For this review, take the finished solid that the model builds, in its own axes (mm). A direction names the side the tool comes from. Coordinates: 2 decimals unless noted, no trailing zeros. Order: outer loops, then holes, each group sorted by start corner. A loop starts at its lowest first (then second) coordinate and runs counter-clockwise, first axis right, second up. Notation, with made-up numbers: M -38,87.25 L 20,87.25 A10 ccw 20,100.25 Z; hole C 5,44 d11. An arc over 180 degrees is marked long. Use one line per item in the form item = value. Start each with the question number.
Solid Edge part; units mm, degrees
sketch "Sketch1" plane through (0, 0, 0) normal (0, -1, 0) x (1, 0, 0)
  line L0 (0, 0) -> (-120, 0)
  line L1 (-120, 0) -> (-120, -10)
  line L2 (-120, -10) -> (-10, -10)
  line L3 (-10, -10) -> (-10, -60)
  line L4 (-10, -60) -> (0, -60)
  line L5 (0, -60) -> (0, 0)
extrude "Protrusion1" add sketch "Sketch1" along normal mid plane 60
sketch "Sketch2" plane through (-42.4264, 0, 42.4264) normal (0.7071068, 0, 0.7071068) x (0, -1, 0)
  line L0 (20, 60) -> (20, 20)
  line L1 (0, 60) -> (20, 60)
  line L2 (-20, 60) -> (0, 60)
  line L3 (-20, 20) -> (-20, 60)
  arc A0 (-20, 20) -> (20, 20) centre (0, 20) ccw
extrude "Protrusion2" add sketch "Sketch2" against normal up to next
sketch "Sketch3" plane through (-21.2132, 0, 21.2132) normal (0.7071068, 0, 0.7071068) x (0, 1, 0)
  circle A0 centre (0, 10.3051) radius 10
extrude "ExtrudedCutout_1" cut sketch "Sketch3" against normal blind 40
sketch "Sketch4" plane through (-28.2843, -20, 14.1421) normal (0, -1, 0) x (1, 0, 0)
  line L0 (10.1152, 4.0269) -> (3.0442, -3.0442)
  line L1 (3.0442, -3.0442) -> (10.1152, -10.1152)
  line L2 (10.1152, -10.1152) -> (17.1863, -3.0442)
  line L3 (17.1863, -3.0442) -> (10.1152, 4.0269)
extrude "Cutout1" cut sketch "Sketch4" against normal up to surface (40 mm away)
sketch "Sketch5" plane through (-60, 0, 0) normal (0, 0, 1) x (1, 0, 0)
  circle A0 centre (-50, -20) radius 5
extrude "Cutout2" cut sketch "Sketch5" against normal up to surface (10 mm away)
sketch "Sketch6" plane through (0, 0, -30) normal (1, 0, 0) x (0, 1, 0)
  circle A0 centre (-20, -20) radius 5
extrude "Cutout3" cut sketch "Sketch6" against normal up to surface (10 mm away)
mirror "Mirror1" about plane through (0, 0, 0) normal (0, -1, 0) of "Cutout2", "Cutout3"
1. The part is to be moulded in two halves that separate along Y. For faces 4 (the flat face through (-36, 0, 36)), 5 (the cylindrical face through (-105.381, 18.085, -4.93)), 6 (the flat face through (-31, 20, 10)), say which applies: pulls with the +Y half, pulls with the -Y half, needs draft (parallel to the pull), parting line crosses it, or undercut.
2. Consider section B-B, the plane z = -50. Write out the cut boundary in (x, y), plus the area to 3 significant figures.
3. Consider section D-D, the plane x = -20. Write out the cut boundary in (y, z), plus the area to 3 significant figures.
4. For pin 1 Ø3 at (x, z) = (-66, 13.5) entering from -Y; pin 2 Ø3 at (x, y) = (-94.5, 23.5) entering from +Z; pin 3 Ø1 at (x, y) = (-13, 19) entering from -Z, all flat-tipped, find the tip position at first contact; note any pin that passes through.
5. To check wall thickness, follow line 1 (Y direction, x = -110, z = -6); line 2 (X direction, y = 20, z = -5.5); line 3 (Z direction, x = -95, y = 27.5). State the ranges of each line that lie inside material, in increasing order.
6. Consider section C-C, the plane x = -110. Write out the cut boundary in (y, z), plus the area to 3 significant figures.
7. Tool access review of faces 1 (the flat face through (-10, 0, -35)), 2 (the flat face through (-21.75, -0.28, 7.61)), 3 (the flat face through (-56.88, 0.14, 0.31)): name each direction out of +Z, -Z, +X, -X, +Y, -Y from which nothing blocks a thin tool from reaching the whole face with its end or side.
8. Consider section A-A, the plane y = -23. Write out the cut boundary in (x, z).
Answers follow:
q1.face_4 = needs draft
q1.face_5 = undercut
q1.face_6 = pulls with the +Y half
q2.outline = M -10,-30 L 0,-30 L 0,-25 L -10,-25 Z; M -10,-15 L 0,-15 L 0,15 L -10,15 Z; M -10,25 L 0,25 L 0,30 L -10,30 Z
q2.area = 400 mm²
q3.outline = M -30,-10 L 30,-10 L 30,0 L 20,0 L 20,5.86 L -20,5.86 L -20,0 L -30,0 Z; M -20,16.34 L 20,16.34 L 20,20 L -20,20 Z
q3.area = 981 mm²
q4.pin_1 = -13.55
q4.pin_2 = 0
q4.pin_3 = -10
q5.line_1 = -30 to -25, -15 to 15, 25 to 30
q5.line_2 = -120 to -115, -105 to 0
q5.line_3 = -10 to 0
q6.outline = M -30,-10 L -25,-10 L -25,0 L -30,0 Z; M -15,-10 L 15,-10 L 15,0 L -15,0 Z; M 25,-10 L 30,-10 L 30,0 L 25,0 Z
q6.area = 400 mm²
q7.face_1 = -Z, -X, +Y, -Y
q7.face_2 = +Y, -Y
q7.face_3 = none
q8.outline = M -120,-10 L -114,-10 L -114,0 L -120,0 Z; M -106,-10 L -10,-10 L -10,-46 L 0,-46 L 0,0 L -106,0 Z; M -10,-60 L 0,-60 L 0,-54 L -10,-54 Z
